Geometry check sheet. Reference: the model listing, model coordinates, mm. A direction names the side the tool comes from. Give positions to 0.01 mm unless a question says otherwise; leave off trailing zeros. Write each loop counter-clockwise with the first axis right and the second up, starting at its lowest first coordinate (ties: lowest second). Pieces come first, ordered by that corner, then holes. Notation, with made-up numbers: M 68.25,-12 L 126.25,-12 A21 ccw 126.25,-5 Z; hole C -12.5,-29 d1. An arc over 180 degrees is marked long. One line per item, written item: value. Start each with the question number.
1. Cross-section at B-B on y = 8.5. Record the cut outline in (x, z), then the cut area to 3 significant figures.
2. Cross-section at A-A on x = 2.75. Record the cut outline in (y, z), then the cut area to 3 significant figures.
3. Gauge pin test, flat end, axial feed: pin 1 (6 mm diameter, centred on x = 9.5, z = 9.5, fed in from +Y). Record the tip position at first contact, or that the pin passes through.
4. Cross-section at C-C on z = 14.75. Record the cut outline in (x, y).
5. Cross-section at D-D on y = 4.75. Record the cut outline in (x, z), then the cut area to 3 significant figures.
6. Tool access check on faces 1 (the face through (6, 3.5, -1)), 2 (the face through (-2, 9, 12)), 3 (the face through (6, 2, 0)). Record the directions out of +Z, -Z, +X, -X, +Y, -Y that give a thin tool (end or side, any length) a straight path to the whole face; none if there is none.
7. Release check for a two-part mould opening along Z. For faces 4 (the face through (0, 10, 11)), 5 (the face through (5, 9, 25.5)), 6 (the face through (6, 6, -1)) record: pulls with the +Z half, pulls with the -Z half, needs draft (parallel to the pull), parting line crosses it, or undercut.
8. Scan lines: line 1 (Z direction, x = 4, y = 2); line 2 (X direction, y = 2, z = 6.75). Record each from-to range of solid material in increasing order.
from build123d import *

# Parameters (mm, degrees)
SKETCH_2_W          = 23.5
SKETCH_2_H          = 18
EXTRUDE_1_DEPTH     = 12.5
SHELL_7_T           = 2
SKETCH_4_W          = 2
SKETCH_4_H          = 2.5
CUT_EXTRUDE_3_DEPTH = 35.734708866
SKETCH_6_W          = 12.5
SKETCH_6_H          = 23.5
CUT_EXTRUDE_4_DEPTH = 35.734708866


with BuildPart() as part:
    # Эскиз2 → Бобышка-Вытянуть1 (new body)
    with BuildSketch(Plane(origin=(0, 0, 0), x_dir=(0, 0, -1), z_dir=(1, 0, 0))):
        with Locations((-11.75, 9)):
            Rectangle(SKETCH_2_W, SKETCH_2_H)
    extrude(amount=EXTRUDE_1_DEPTH)

    # Оболочка7
    shell_7_openings = [part.faces().sort_by_distance(p)[0] for p in [
        (12.5, 9, 11.75),
    ]]
    offset(amount=SHELL_7_T, openings=shell_7_openings, kind=Kind.INTERSECTION)

    # Эскиз4 → Вырез-Вытянуть3 (cut, through all)
    with BuildSketch(Plane(origin=(0, 0, 0), x_dir=(0, 0, -1), z_dir=(1, 0, 0))):
        with Locations((1, 4.75)):
            Rectangle(SKETCH_4_W, SKETCH_4_H)
    extrude(amount=CUT_EXTRUDE_3_DEPTH, mode=Mode.SUBTRACT)

    # Эскиз6 → Вырез-Вытянуть4 (cut, through all)
    with BuildSketch(Plane.XZ.offset(-18)):
        with Locations((6.25, 11.75)):
            Rectangle(SKETCH_6_W, SKETCH_6_H)
    extrude(amount=-CUT_EXTRUDE_4_DEPTH, mode=Mode.SUBTRACT)


solid = part.part
Report:
1. outline: M -2,-2 L 12.5,-2 L 12.5,0 L 0,0 L 0,23.5 L 12.5,23.5 L 12.5,25.5 L -2,25.5 Z
1. area: 105 mm^2
2. outline: M -2,-2 L 3.5,-2 L 3.5,0 L 0,0 L 0,23.5 L 20,23.5 L 20,25.5 L -2,25.5 Z; M 6,-2 L 20,-2 L 20,0 L 6,0 Z
2. area: 130 mm^2
3. pin 1: stops at y = 0
4. outline: M -2,-2 L 12.5,-2 L 12.5,0 L 0,0 L 0,20 L -2,20 Z
5. outline: M -2,-2 L 0,-2 L 0,23.5 L 12.5,23.5 L 12.5,25.5 L -2,25.5 Z
5. area: 80.0 mm^2
6. face 1: -Z, +X
6. face 2: +Z, -Z, -X, +Y, -Y
6. face 3: +X, +Y
7. face 4: undercut
7. face 5: pulls with the +Z half
7. face 6: needs draft
8. line 1: z = -2 to 0, 23.5 to 25.5
8. line 2: x = -2 to 0
